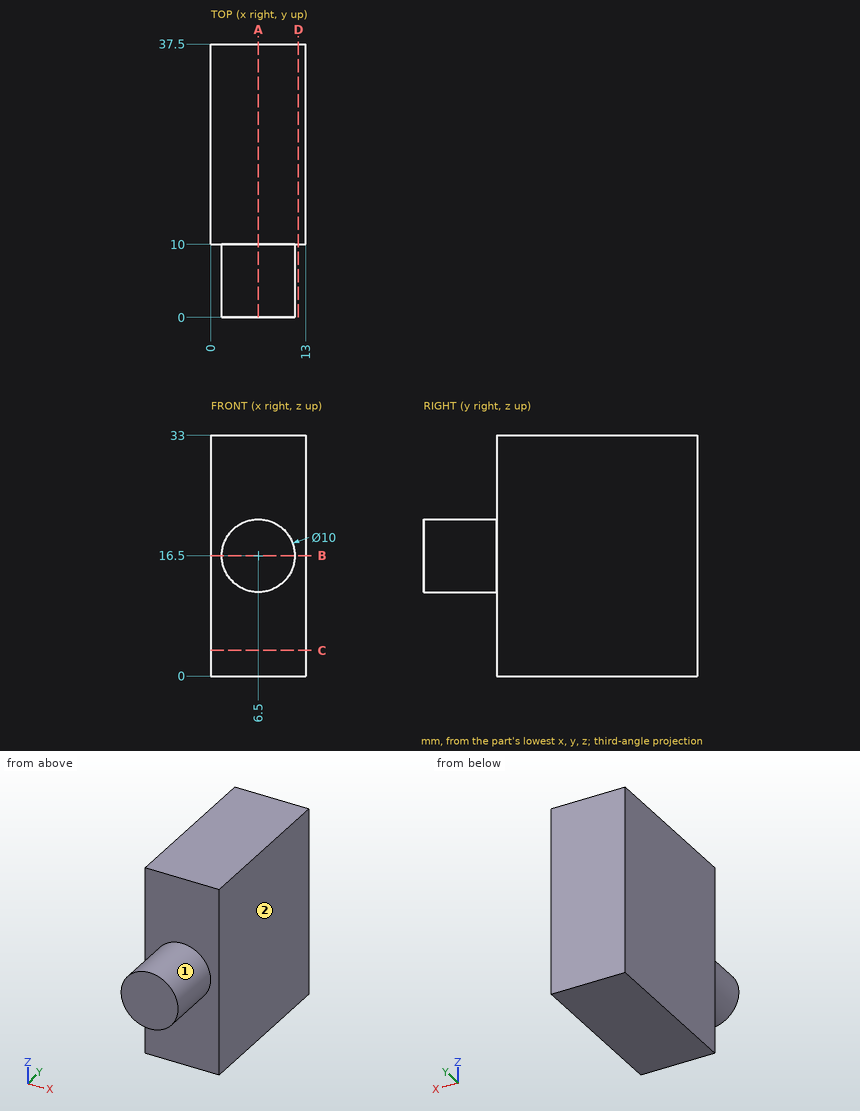
Check sheet for the drawn part. Datum: minimum x, y, z corner. Units: mm. A direction names the side the tool comes from. Give positions to 0.01 mm unless a question says otherwise; leave off trailing zeros. Write each loop counter-clockwise with the first axis right and the second up, starting at its lowest first coordinate (ties: lowest second). Pieces come first, ordered by that corner, then holes. Notation, with made-up numbers: M -6.75,37 L 25.25,37 A32 ccw 25.25,68 Z; hole C -30.5,-27.5 d9. An arc over 180 degrees is marked long. One line per question, with ' | ' between items.
1) Section check D-D on x = 12. Enter the section's corners in (y, z).
Result:
outline: M 10,0 L 37.5,0 L 37.5,33 L 10,33 Z
2) Section check C-C on z = 3.5. Enter the section's corners in (x, y).
Result:
outline: M 0,10 L 13,10 L 13,37.5 L 0,37.5 Z
3) Set-up check for the marked faces 1 and 2: record each of +Z, -Z, +X, -X, +Y, -Y from which the full face is reachable in a straight line by a thin tool's end or side.
Result:
face 1: -Y | face 2: +Z, -Z, +X, +Y, -Y
4) Section check B-B on z = 16.5. Enter the section's corners in (x, y).
Result:
outline: M 0,10 L 1.5,10 L 1.5,0 L 11.5,0 L 11.5,10 L 13,10 L 13,37.5 L 0,37.5 Z
5) Section check A-A on x = 6.5. Enter the section's corners in (y, z), plus the area to 3 significant figures.
Result:
outline: M 0,11.5 L 10,11.5 L 10,0 L 37.5,0 L 37.5,33 L 10,33 L 10,21.5 L 0,21.5 Z | area: 1,010 mm2
6) Thickness scan on line 1 along Y through (x, z) = (12, 23.5); line 2 along X through (y, z) = (6, 16.5); line 3 along Z through (x, y) = (10.25, 9). Record the ranges inside material, lowest first. Write a range as [from, to].
Result:
line 1: y = [10, 37.5] | line 2: x = [1.5, 11.5] | line 3: z = [13.19, 19.81]
7) Gauge pin test, flat end, axial feed: pin 1 Ø4 at (x, z) = (3.5, 9.5) entering from -Y. Record the tip position at first contact, or that the pin passes through.
Result:
pin 1: stops at y = 10
